from build123d import *

# Parameters (mm, degrees)
SKETCH_R              = 29.5
PAD_DEPTH             = 11.5
SKETCH001_R           = 26.5
POCKET_DEPTH          = 11.501
PAD001_DEPTH          = 10
POLARPATTERN_COUNT    = 5
SKETCH003_R           = 14
SKETCH003_R_2         = 3.6
PAD002_DEPTH          = 10
SKETCH004_W           = 14
SKETCH004_H           = 14
POCKET001_DEPTH       = 5.75
SKETCH005_R           = 11.3
POCKET002_DEPTH       = 4
POCKET003_DEPTH       = 179.9557416964
POLARPATTERN001_COUNT = 30


with BuildPart() as part:
    # Sketch → Pad (new body)
    with BuildSketch(Plane.XZ):
        Circle(SKETCH_R)
    extrude(amount=PAD_DEPTH)

    # Sketch001 (on Face3 of Pad) → Pocket (cut, through all)
    with BuildSketch(Plane.XZ.offset(11.5)):
        Circle(SKETCH001_R)
    extrude(amount=-POCKET_DEPTH, mode=Mode.SUBTRACT)

    # Sketch002 → Pad001 (join)
    with BuildSketch(Plane.XZ):
        with BuildLine():
            ThreePointArc((1, 13.9642400438), (0, 14), (-1, 13.9642400438))
            Line((-1, 13.9642400438), (-1, 26.4811253537))
            ThreePointArc((1, 26.4811253537), (0, 26.5), (-1, 26.4811253537))
            Line((1, 13.9642400438), (1, 26.4811253537))
        make_face()
    pad001 = extrude(amount=PAD001_DEPTH)

    # PolarPattern: Pad001 ×5 about axis
    polarpattern_axis = Axis((0, 0, 0), (0, -1, 0))
    for i in range(1, POLARPATTERN_COUNT):
        add(pad001.rotate(polarpattern_axis, i * 360 / POLARPATTERN_COUNT))

    # Sketch003 → Pad002 (join)
    with BuildSketch(Plane.XZ):
        Circle(SKETCH003_R)
        Circle(SKETCH003_R_2, mode=Mode.SUBTRACT)
    extrude(amount=PAD002_DEPTH)

    # Sketch004 (on Face2 of Pad002) → Pocket001 (cut)
    with BuildSketch(Plane(origin=(0, 0, 0), x_dir=(1, 0, 0), z_dir=(0, 1, 0))):
        Rectangle(SKETCH004_W, SKETCH004_H)
    extrude(amount=-POCKET001_DEPTH, mode=Mode.SUBTRACT)

    # Sketch005 (on Face2 of Pocket001) → Pocket002 (cut)
    with BuildSketch(Plane(origin=(0, 0, 0), x_dir=(1, 0, 0), z_dir=(0, 1, 0))):
        Circle(SKETCH005_R)
    extrude(amount=-POCKET002_DEPTH, mode=Mode.SUBTRACT)

    # Sketch006 (on Face34 of Pocket002) → Pocket003 (cut, through all)
    with BuildSketch(Plane.XZ.offset(11.5)):
        with BuildLine():
            Line((-1.03, 29.4820131606), (-1.03, 28.4813816379))
            ThreePointArc((1.03, 28.4813816378), (0, 28.5), (-1.03, 28.4813816378))
            Line((1.03, 29.4820131606), (1.03, 28.4813816378))
            ThreePointArc((1.03, 29.4820131606), (0, 29.5), (-1.03, 29.4820131606))
        make_face()
    pocket003 = extrude(amount=-POCKET003_DEPTH, mode=Mode.SUBTRACT)

    # PolarPattern001: Pocket003 ×30 about axis
    polarpattern001_axis = Axis((0, -11.5, 0), (0, -1, 0))
    for i in range(1, POLARPATTERN001_COUNT):
        add(pocket003.rotate(polarpattern001_axis, i * 360 / POLARPATTERN001_COUNT), mode=Mode.SUBTRACT)


solid = part.part
Input: part model. Units: mm. Frame: model coordinates. A direction names the side the tool comes from. Coordinates: 2 decimals unless noted, no trailing zeros. Loops run counter-clockwise (first coordinate to the right, second up) from the corner with the lowest first, then second, coordinate; pieces in that order, holes last.
Q1. Cut plane C-C (y = -2). Give the number of separate pieces and of enclosed holes in the cut face, then the cut area to 3 significant figures.
Q2. Draft query along X for faces 1 (the face through (-8.14, -4.93, 11.39)), 2 (the face through (-5.91, -5.83, 27.88)), 3 (the face through (-26.938, -5.67, 12.025)), 4 (the face through (26.961, -5.67, 11.972)). Return one class per face: +X half, -X half, draft (parallel to the pull), parting line (faces both ways), or undercut.
Q3. Material intervals for line 1 (X direction, y = -7.5, z = 0); line 2 (X direction, y = -3.5, z = 0); line 3 (X direction, y = -7.5, z = 17), sorted ascending.
Q4. Cut plane B-B (x = 0). Output: boundary loops of the cut face in (y, z), then the cut area to 4 significant figures.
Q5. Cut plane D-D (x = -6). Output: boundary loops of the cut face in (y, z), then the cut area to 3 significant figures.
Q6. Contact query for flat-ended pins moving along their axis: pin 1 (1 mm diameter, centred on y = -5, z = 22, fed in from -X); pin 2 (0.9 mm diameter, centred on y = -4.5, z = -3, fed in from -X); pin 3 (6 mm diameter, centred on x = -12, z = -14, fed in from -Y). Output: stop coordinate, or through.
Q7. Set-up query: faces 5 (the face through (-29.5, -5.7, 0)), 6 (the face through (11.03, -4.93, -16.88)), 7 (the face through (7, -5, 0)). Return all of +Z, -Z, +X, -X, +Y, -Y with unobstructed straight access to the full face (end or side cutting, diameter ignored); none if empty.
Q8. Cut plane A-A (z = 0). Output: boundary loops of the cut face in (x, y).
Working result:
1. separate pieces: 1
1. enclosed holes: 6
1. area: 806 mm2
2. face 1: undercut
2. face 2: undercut
2. face 3: -X half
2. face 4: +X half
3. line 1: x = -29.5 to -26.5, -14 to -3.6, 3.6 to 14, 26.5 to 29.5
3. line 2: x = -29.5 to -26.5, -14 to -11.3, 11.3 to 14, 26.5 to 29.5
3. line 3: x = -24.11 to -20.33, -1 to 1, 20.33 to 24.11
4. outline: (-11.5, -28.5) - (0, -28.5) - (0, -26.5) - (-11.5, -26.5) - close; (-11.5, 26.5) - (-10, 26.5) - (-10, 3.6) - (-5.75, 3.6) - (-5.75, 7) - (-4, 7) - (-4, 11.3) - (0, 11.3) - (0, 28.5) - (-11.5, 28.5) - close; (-10, -14) - (0, -14) - (0, -11.3) - (-4, -11.3) - (-4, -7) - (-5.75, -7) - (-5.75, -3.6) - (-10, -3.6) - close
4. area: 305.5 mm2
5. outline: (-11.5, -27.86) - (0, -27.86) - (0, -25.81) - (-11.5, -25.81) - close; (-11.5, 25.81) - (0, 25.81) - (0, 27.86) - (-11.5, 27.86) - close; (-10, -12.65) - (0, -12.65) - (0, -9.58) - (-4, -9.58) - (-4, -7) - (-5.75, -7) - (-5.75, 7) - (-4, 7) - (-4, 9.58) - (0, 9.58) - (0, 12.65) - (-10, 12.65) - close
5. area: 199 mm2
6. pin 1: stops at x = -20.2
6. pin 2: stops at x = -28.39
6. pin 3: stops at y = -10
7. face 5: -X, +Y, -Y
7. face 6: +Y, -Y
7. face 7: +Y
8. outline: (-29.5, -11.5) - (-26.5, -11.5) - (-26.5, 0) - (-29.5, 0) - close; (-14, -10) - (-3.6, -10) - (-3.6, -5.75) - (-7, -5.75) - (-7, -4) - (-11.3, -4) - (-11.3, 0) - (-14, 0) - close; (3.6, -10) - (14, -10) - (14, 0) - (11.3, 0) - (11.3, -4) - (7, -4) - (7, -5.75) - (3.6, -5.75) - close; (26.5, -11.5) - (29.5, -11.5) - (29.5, 0) - (26.5, 0) - close
